Job drawing, mm, ordinate dimensions from the low corner. One solid piece. A direction names the side the tool comes from. Round coordinates to 2 decimals unless told otherwise and drop trailing zeros. Write each loop counter-clockwise with the first axis right and the second up, starting at its lowest first coordinate (ties: lowest second). Pieces come first, ordered by that corner, then holes.
1) Saw through at D-D (y = 8.5). Write the cut outline in (x, z).
2) Pull direction Y, two halves, no side cores. Call the marked faces 5, 6 and 7: +Y half, -Y half, draft (parallel to the pull), parting line (faces both ways), or undercut.
3) Saw through at C-C (z = 3.5). Write the cut outline in (x, y), plus the area to 3 significant figures.
4) Which spindle directions (+Z, -Z, +X, -X, +Y, -Y) get a long thin tool onto all of the face, cutting with end or side? Do the marked faces 1, 2, 3 and 4. Say none if no direction does.
5) Saw through at B-B (x = 4.5). Write the cut outline in (y, z).
6) Flat gauge pins, fed straight in: pin 1 (1.5 mm diameter, centred on x = 8, z = 1.5, fed in from +Y); pin 2 (0.6 mm diameter, centred on x = 0.5, z = 3.5, fed in from -Y); pin 3 (0.9 mm diameter, centred on x = 0.5, y = 13.5, fed in from +Z); pin 4 (0.8 mm diameter, centred on x = 3.5, z = 1, fed in from -Y). Where does each tip first touch, or does it go through?
7) Wall check: probe 1 along Y at (x, z) = (2.25, 2); probe 2 along Z at (x, y) = (8.5, 15.25); probe 3 along X at (y, z) = (15.75, 5). Give the ranges that are in metal, low to high.
8) Saw through at A-A (y = 16.75). Write the cut outline in (x, z), plus the area to 3 significant figures.
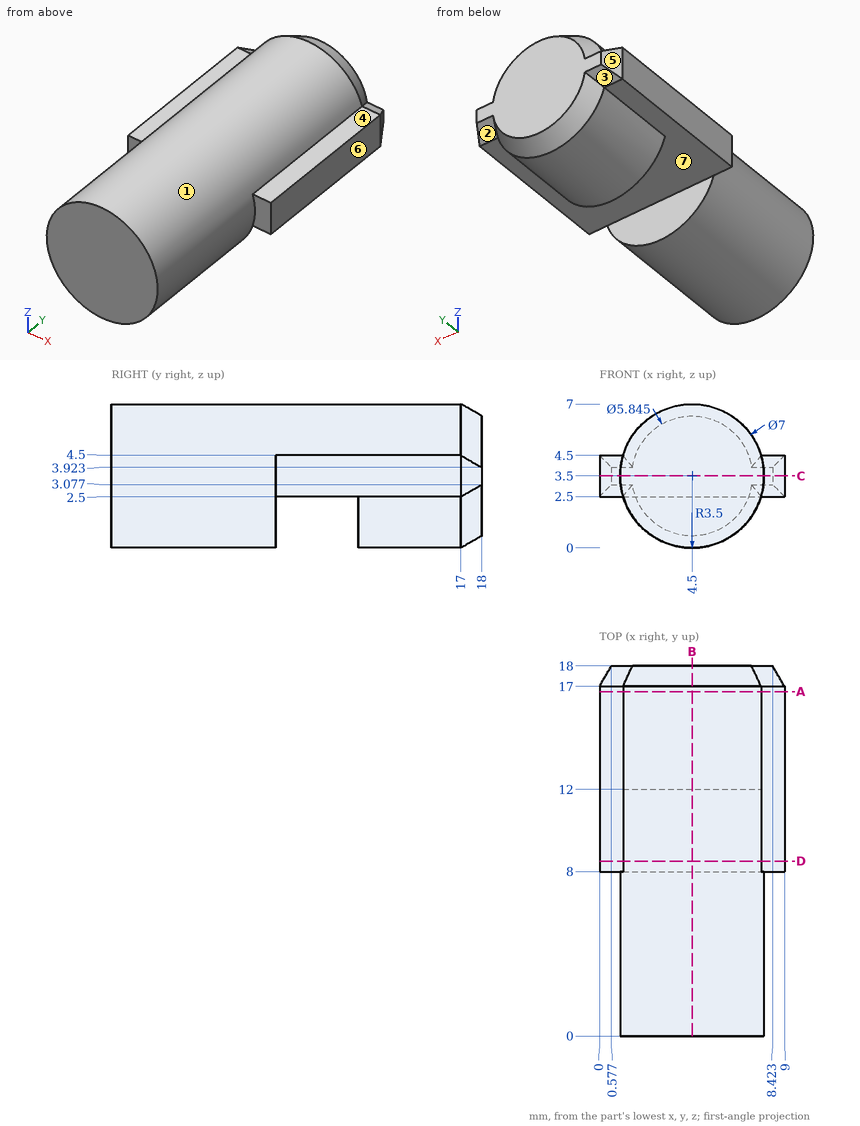
Evaluation:
1. outline: (0, 2.5) - (9, 2.5) - (9, 4.5) - (7.85, 4.5) arc R3.5 ccw to (1.15, 4.5) - (0, 4.5) - close
2. face 5: +Y half
2. face 6: draft
2. face 7: undercut
3. outline: (0, 8) - (1, 8) - (1, 0) - (8, 0) - (8, 8) - (9, 8) - (9, 17) - (8.42, 18) - (0.58, 18) - (0, 17) - close
3. area: 145 mm2
4. face 1: -Y
4. face 2: -Z, +X, +Y
4. face 3: -Z, -X, +Y
4. face 4: +Z, +X, +Y, -Y
5. outline: (0, 0) - (8, 0) - (8, 2.5) - (12, 2.5) - (12, 0) - (17, 0) - (18, 0.58) - (18, 6.42) - (17, 7) - (0, 7) - close
6. pin 1: stops at y = 17.38
6. pin 2: stops at y = 8
6. pin 3: stops at z = 4.5
6. pin 4: stops at y = 0
7. probe 1: y = 0 to 8, 12 to 18
7. probe 2: z = 2.5 to 4.5
7. probe 3: x = 1.34 to 7.66
8. outline: (0, 2.5) - (1.15, 2.5) arc R3.5 ccw to (7.85, 2.5) - (9, 2.5) - (9, 4.5) - (7.85, 4.5) arc R3.5 ccw to (1.15, 4.5) - (0, 4.5) - close
8. area: 42.7 mm2
